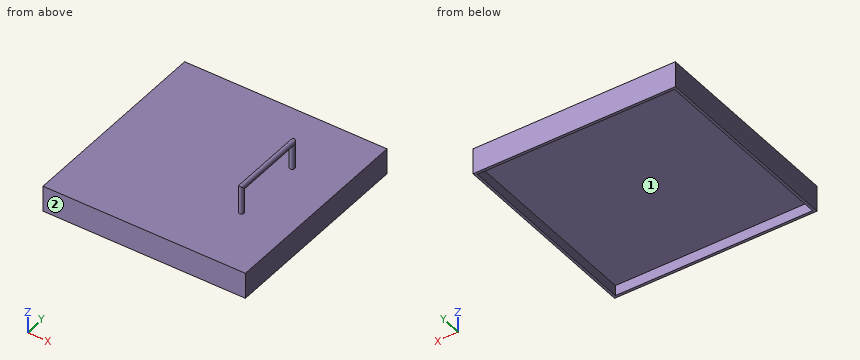
```python
from build123d import *

# Parameters (mm, degrees)
F0_W     = 390
F0_H     = 390
F1_DEPTH = 50
F2_W     = 380
F2_H     = 380
F3_DEPTH = 20
F6_R     = 5


with BuildPart() as f1:
    # F0 (on Top) → F1 (new body)
    with BuildSketch(Plane.XY):
        Rectangle(F0_W, F0_H)
    extrude(amount=F1_DEPTH)

    # F2 (on face) → F3 (cut)
    with BuildSketch(Plane(origin=(0, 0, 0), x_dir=(1, 0, 0), z_dir=(0, 0, -1))):
        Rectangle(F2_W, F2_H)
    extrude(amount=-F3_DEPTH, mode=Mode.SUBTRACT)

    # F7: sweep along a path in F5
    with BuildLine(Plane.YZ.offset(100)) as f7_path:
        Line((70, 50), (70, 100))
        Line((70, 100), (-70, 100))
        Line((-70, 100), (-70, 50))
    # F6 (on face) → F7 (sweep)
    with BuildSketch(Plane.XY.offset(50)):
        with Locations((100, 70)):
            Circle(F6_R)
    sweep(path=f7_path.line, transition=Transition.RIGHT)


solid = f1.part
```
Part model, mm, in its own coordinate system. Face numbers are marked on the shaded views. A direction names the side the tool comes from. Round coordinates to 2 decimals unless told otherwise and drop trailing zeros. Loops run counter-clockwise (first coordinate to the right, second up) from the corner with the lowest first, then second, coordinate; pieces in that order, holes last.
1. Slice it at C-C (x = -14.5). Give the cut face in (y, z), and give its area (3 significant figures).
Solutions:
outline: (-195, 0) - (-190, 0) - (-190, 20) - (190, 20) - (190, 0) - (195, 0) - (195, 50) - (-195, 50) - close
area: 11,900 mm2
2. Slice it at B-B (z = 11.5). Give the cut face in (x, y), and give its area (3 significant figures).
Solutions:
outline: (-195, -195) - (195, -195) - (195, 195) - (-195, 195) - close; hole (-190, -190) - (190, -190) - (190, 190) - (-190, 190) - close
area: 7,700 mm2
3. Slice it at A-A (y = 48). Give the cut face in (x, z), and give its area (3 significant figures).
Solutions:
outline: (-195, 0) - (-190, 0) - (-190, 20) - (190, 20) - (190, 0) - (195, 0) - (195, 50) - (-195, 50) - close; circle Ø10 at (100, 100)
area: 12,000 mm2
4. 3-axis set-ups, long thin cutter, end or side, ignore diameter. For the marked faces 1 and 2: which of +Z, -Z, +X, -X, +Y, -Y reach the whole face in a straight line?
Solutions:
face 1: -Z
face 2: +Z, -Z, +X, -X, -Y
5. Drill centre lines: line 1 along Y through (x, z) = (-127, 12.5); line 2 along Z through (x, y) = (-136.5, -124). Where is each one in solid material? Low to high.
Solutions:
line 1: y = -195 to -190, 190 to 195
line 2: z = 20 to 50
6. Slice it at D-D (z = 74). Give the cut face in (x, y).
Solutions:
outline: circle Ø10 at (100, -70); circle Ø10 at (100, 70)
7. Flat gauge pins, fed straight in: pin 1 (4 mm diameter, centred on x = -144, y = 28, fed in from -Z); pin 2 (4 mm diameter, centred on x = -136.5, y = 100, fed in from +Z). Where does each tip first touch, or does it go through?
Solutions:
pin 1: stops at z = 20
pin 2: stops at z = 50
